Check sheet for the modelled part. Datum: model origin and axes. Units: mm. Face numbers are marked on the shaded views. A direction names the side the tool comes from. Round coordinates to 2 decimals unless told otherwise and drop trailing zeros. Order: outer loops, then holes, each group sorted by start corner. A loop starts at its lowest first (then second) coordinate and runs counter-clockwise, first axis right, second up. Notation, with made-up numbers: (74, 47.5) -> (126, 47.5) arc R30 ccw to (126, 77.5) -> close; hole circle Ø7 at (87, 69.5). An arc over 180 degrees is marked (long way). Use CSV: the item, a comma, the result in double quotes.
```python
from build123d import *

# Parameters (mm, degrees)
SKETCH1_W           = 88
SKETCH1_H           = 47
SKETCH1_R           = 2.5
BOSS_EXTRUDE1_DEPTH = 60
BOSS_EXTRUDE2_START = 20
SKETCH1_2_R         = 2.5
BOSS_EXTRUDE2_DEPTH = 40
SKETCH2_W           = 9.5
SKETCH2_H           = 47
BOSS_EXTRUDE3_DEPTH = 24.5
FILLET1_R           = 3


with BuildPart() as part:
    # Sketch1 → Boss-Extrude1 (new body)
    with BuildSketch(Plane(origin=(0, 0, 0), x_dir=(1, 0, 0), z_dir=(0, 1, 0))):
        Rectangle(SKETCH1_W, SKETCH1_H)
        with Locations(Location((25.5, 18, 0), (0, 0, 270))):
            Circle(SKETCH1_R, mode=Mode.SUBTRACT)
        with Locations(Location((25.5, -18, 0), (0, 0, 90))):
            Circle(SKETCH1_R, mode=Mode.SUBTRACT)
    extrude(amount=BOSS_EXTRUDE1_DEPTH)

    # Sketch1_2 → Boss-Extrude2 (add)
    with BuildSketch(Plane(origin=(0, 0, 0), x_dir=(1, 0, 0), z_dir=(0, 1, 0)).offset(BOSS_EXTRUDE2_START)):
        with Locations(Location((25.5, -18, 0), (0, 0, 90))):
            Circle(SKETCH1_2_R)
        with Locations(Location((25.5, 18, 0), (0, 0, 270))):
            Circle(SKETCH1_2_R)
    extrude(amount=BOSS_EXTRUDE2_DEPTH)

    # Sketch2 → Boss-Extrude3 (add)
    with BuildSketch(Plane(origin=(0, 60, 0), x_dir=(1, 0, 0), z_dir=(0, 1, 0))):
        with Locations((39.25, 0)):
            Rectangle(SKETCH2_W, SKETCH2_H)
    extrude(amount=BOSS_EXTRUDE3_DEPTH)

    # Fillet1
    fillet1_edges = [part.edges().sort_by_distance(p)[0] for p in [
        (34.5, 60, 0),
    ]]
    fillet(fillet1_edges, radius=FILLET1_R)


solid = part.part
```
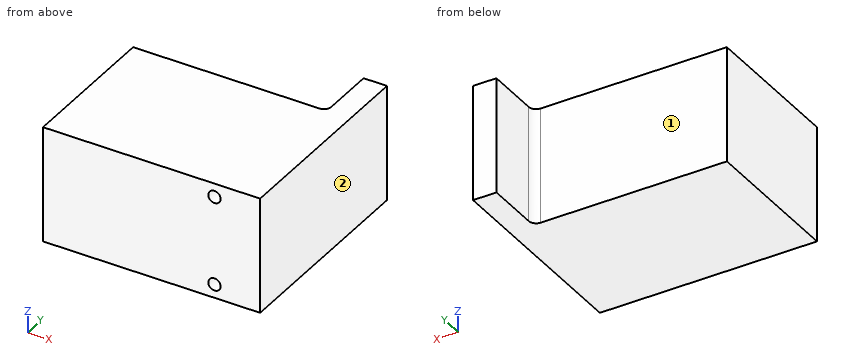
Q1. Sectioned sample at D-D, the plane z = -18. Enter the section's corners in (x, y), then the cut area to 3 significant figures.
Result sheet:
outline,"(-44, 0) -> (23, 0) -> (23, 20) -> (28, 20) -> (28, 0) -> (44, 0) -> (44, 84.5) -> (34.5, 84.5) -> (34.5, 63) arc R3 cw to (31.5, 60) -> (-44, 60) -> close"
area,"5,410 mm^2"
Q2. Go/stop test with flat-tipped pins: pin 1 (17 mm diameter, centred on y = 78.5, z = 9.5, fed in from -X); pin 2 (4 mm diameter, centred on y = 63.5, z = 1, fed in from -X); pin 3 (1 mm diameter, centred on x = -28, z = -13, fed in from +Y). Record where each tip stops, or that it passes through.
Result sheet:
pin 1,"stops at x = 34.5"
pin 2,"stops at x = 34.1"
pin 3,"stops at y = 60"
Q3. Sectioned sample at B-B, the plane x = 25.5. Enter the section's corners in (y, z), then the cut area to 3 significant figures.
Result sheet:
outline,"(0, -23.5) -> (60, -23.5) -> (60, 23.5) -> (0, 23.5) -> (0, 20.5) -> (20, 20.5) -> (20, 15.5) -> (0, 15.5) -> (0, -15.5) -> (20, -15.5) -> (20, -20.5) -> (0, -20.5) -> close"
area,"2,620 mm^2"
Q4. Access from +Z, -Z, +X, -X, +Y, -Y to the whole of each face (thin tool, end or side, straight path). Record for the marked faces 1 and 2.
Result sheet:
face 1,"+Z, -Z, -X, +Y"
face 2,"+Z, -Z, +X, +Y, -Y"
Q5. Scan lines: L1, parallel to Z at x = 25, y = 15; L2, parallel to X at y = 8, z = -18; L3, parallel to X at y = 64, z = -11.5. Record each from-to range of solid material in increasing order.
Result sheet:
L1,"z = -23.5 to -20.45, -15.55 to 15.55, 20.45 to 23.5"
L2,"x = -44 to 23, 28 to 44"
L3,"x = 34.5 to 44"
Q6. Sectioned sample at A-A, the plane z = 3. Enter the section's corners in (x, y), then the cut area to 3 significant figures.
Result sheet:
outline,"(-44, 0) -> (44, 0) -> (44, 84.5) -> (34.5, 84.5) -> (34.5, 63) arc R3 cw to (31.5, 60) -> (-44, 60) -> close"
area,"5,510 mm^2"
Q7. Sectioned sample at C-C, the plane y = 72. Enter the section's corners in (x, z).
Result sheet:
outline,"(34.5, -23.5) -> (44, -23.5) -> (44, 23.5) -> (34.5, 23.5) -> close"
